Verification items for the finished model (mm, model axes). Face numbers are marked on the shaded views. A direction names the side the tool comes from. Coordinates: 2 decimals unless noted, no trailing zeros. Order: outer loops, then holes, each group sorted by start corner. A loop starts at its lowest first (then second) coordinate and runs counter-clockwise, first axis right, second up. Notation, with made-up numbers: M -24.75,-40 L 13.25,-40 A13 ccw 13.25,-36 Z; hole C 47,60 d6. An arc over 180 degrees is marked long. Write item = value, one per line.
Autodesk Inventor part; units mm, degrees
ref_plane "YZ Plane" through (0, 0, 0) normal (1, 0, 0) x (0, 1, 0)
ref_plane "XZ Plane" through (0, 0, 0) normal (0, 1, 0) x (-1, 0, 0)
ref_plane "XY Plane" through (0, 0, 0) normal (0, 0, 1) x (1, 0, 0)
sketch "Sketch1" plane through (0, 0, 0) normal (1, 0, 0) x (0, 1, 0)
  line L0 (-6, -12.5) -> (-6, -12.9)
  arc A0 (-6, -12.9) -> (-5.6, -13.3) centre (-5.6, -12.9) ccw
  line L1 (-5.6, -13.3) -> (-4.9, -13.3)
  arc A1 (-4.9, -13.3) -> (-4.7, -13.1) centre (-4.9, -13.1) ccw
  line L2 (-4.7, -13.1) -> (-4.7, -12.85)
  arc A2 (-4.5, -12.65) -> (-4.7, -12.85) centre (-4.5, -12.85) ccw
  line L3 (-4.5, -12.65) -> (-1.8, -12.65)
  arc A3 (-1.4, -13.05) -> (-1.8, -12.65) centre (-1.8, -13.05) ccw
  line L4 (-1.4, -13.05) -> (-1.4, -18.75)
  line L5 (-1.8, -19.15) -> (-4.5, -19.15)
  arc A4 (-1.8, -19.15) -> (-1.4, -18.75) centre (-1.8, -18.75) ccw
  arc A5 (-4.7, -18.95) -> (-4.5, -19.15) centre (-4.5, -18.95) ccw
  line L6 (-4.7, -18.95) -> (-4.7, -18.7)
  arc A6 (-4.7, -18.7) -> (-4.9, -18.5) centre (-4.9, -18.7) ccw
  line L7 (-4.9, -18.5) -> (-5.6, -18.5)
  arc A7 (-5.6, -18.5) -> (-6, -18.9) centre (-5.6, -18.9) ccw
  line L8 (-6, -18.9) -> (-6, -19.5)
  line L9 (-6.5, -6.5) -> (-6.5, -12.5)
  line L10 (-6.5, -12.5) -> (-2.5, -12.5)
  line L11 (-1.05, -19.5) -> (-6.5, -19.5)
  line L12 (-6.5, -19.5) -> (-6.5, -26)
  line L13 (-6.5, -26) -> (-1.05, -26)
  line L14 (-6, -26) -> (-6, -26.6)
  arc A8 (-6, -26.6) -> (-5.6, -27) centre (-5.6, -26.6) ccw
  line L15 (-5.6, -27) -> (-4.9, -27)
  arc A9 (-4.9, -27) -> (-4.7, -26.8) centre (-4.9, -26.8) ccw
  arc A10 (-4.5, -26.35) -> (-4.7, -26.55) centre (-4.5, -26.55) ccw
  line L16 (-4.7, -26.8) -> (-4.7, -26.55)
  line L17 (-4.5, -26.35) -> (-1.8, -26.35)
  arc A11 (-1.4, -26.75) -> (-1.8, -26.35) centre (-1.8, -26.75) ccw
  line L18 (-1.4, -26.75) -> (-1.4, -32.45)
  arc A12 (-1.8, -32.85) -> (-1.4, -32.45) centre (-1.8, -32.45) ccw
  line L19 (-1.8, -32.85) -> (-4.5, -32.85)
  arc A13 (-4.7, -32.65) -> (-4.5, -32.85) centre (-4.5, -32.65) ccw
  line L20 (-4.7, -32.65) -> (-4.7, -32.4)
  arc A14 (-4.7, -32.4) -> (-4.9, -32.2) centre (-4.9, -32.4) ccw
  line L21 (-4.9, -32.2) -> (-5.6, -32.2)
  arc A15 (-5.6, -32.2) -> (-6, -32.6) centre (-5.6, -32.6) ccw
  line L22 (-6, -32.6) -> (-6, -33)
  line L23 (-2.5, -33) -> (-6.5, -33)
  line L24 (-6.5, -33) -> (-6.5, -39)
  line L25 (32.5, 0) -> (0, 0)
  circle A16 centre (0, -6.5) radius 4.75
  circle A17 centre (32.5, -6.5) radius 4.75
  circle A18 centre (0, -39) radius 4.75
  circle A19 centre (32.5, -39) radius 4.75
  line L26 (39, -26) -> (39, -19.5)
  line L27 (39, -12.5) -> (39, -6.5)
  line L28 (39, -39) -> (39, -33)
  line L29 (26.5, -45.5) -> (32.5, -45.5)
  line L30 (0, -45.5) -> (6, -45.5)
  line L31 (13, -45.5) -> (19.5, -45.5)
  circle A20 centre (16.25, -22.75) radius 15
  circle A21 centre (16.2588, 5.0016) radius 2.5
  circle A22 centre (16.25, -50.5) radius 2.5
  circle A23 centre (16.25, -22.75) radius 5
  circle A24 centre (16.25, -22.75) radius 8.45
  line L32 (24.75, -27.6575) -> (24.75, -17.8425)
  line L33 (44, 10) -> (-11.5, 10)
  line L34 (-11.5, 10) -> (-11.5, -55.5)
  line L35 (-11.5, -55.5) -> (44, -55.5)
  line L36 (44, -55.5) -> (44, 10)
  line L37 (-11.5, 30) -> (44, 30)
  line L38 (-11.5, -75.5) -> (-11.5, 30)
  line L39 (44, 30) -> (44, -75.5)
  line L40 (44, -75.5) -> (-11.5, -75.5)
  circle A25 centre (16.25, -65.5) radius 5
  circle A26 centre (16.25, 20) radius 5
  line L41 (44, 30) -> (44, 50)
  line L42 (44, -75.5) -> (44, -95.5)
  line L43 (110, 50) -> (84, 50)
  line L44 (84, 50) -> (84, -95.5)
  line L45 (84, -95.5) -> (110, -95.5)
  line L46 (110, -95.5) -> (110, 50)
  line L47 (84, 50) -> (104, 50)
  line L48 (104, -95.5) -> (84, -95.5)
  line L49 (84, -95.5) -> (84, 50)
  line L50 (84, 50) -> (64, 50)
  line L51 (64, 50) -> (64, -95.5)
  line L52 (64, -95.5) -> (84, -95.5)
  line L53 (84, -95.5) -> (84, 50)
  line L54 (64, 50) -> (44, 50)
  line L55 (44, 50) -> (44, -95.5)
  line L56 (44, -95.5) -> (64, -95.5)
  line L57 (64, -95.5) -> (64, 50)
  line L58 (44, 30) -> (54, 30)
  line L59 (100.8097, 50) -> (100.8097, 40)
  line L60 (94, -95.5) -> (94, -85.5)
  line L61 (110, 40) -> (54, 40)
  line L62 (54, 40) -> (54, -85.5)
  line L63 (54, -85.5) -> (110, -85.5)
  line L64 (110, 50) -> (136, 50)
  line L65 (136, 50) -> (136, 40)
  line L66 (136, 40) -> (110, 40)
  line L67 (110, -85.5) -> (136, -85.5)
  line L68 (136, -85.5) -> (136, -95.5)
  line L69 (136, -95.5) -> (110, -95.5)
  dimension "d0" = 20
  dimension "d1" = 20
  dimension "d2" = 55.5
  dimension "d3" = 26
  dimension "d5" = 20
  dimension "d6" = 45.5
  dimension "d7" = 20
  dimension "d8" = 10
  dimension "d9" = 10
  dimension "d10" = 26
extrude "Extrusion1" add sketch "Sketch1" along normal blind 75.5 contours L39 L58 L62 L63 L51 L56 L42 L36 | L41 L54 L51 L61 L62 L58 | L50 L44 L61 L51 | L51 L63 L44 L52 | L43 L59 L61 L44 | L44 L63 L60 L45 | L43 L46 L61 L59 | L60 L63 L46 L45 | L64 L65 L66 L46 | L67 L68 L69 L46
sketch "Sketch2" plane through (0, 44, -95.5) normal (0, -1, 0) x (1, 0, 0)
  line L0 (15.5, 83) -> (15.5, 82.6)
  arc A0 (15.5, 82.6) -> (15.9, 82.2) centre (15.9, 82.6) ccw
  line L1 (15.9, 82.2) -> (16.6, 82.2)
  arc A1 (16.6, 82.2) -> (16.8, 82.4) centre (16.6, 82.4) ccw
  line L2 (16.8, 82.4) -> (16.8, 82.65)
  arc A2 (17, 82.85) -> (16.8, 82.65) centre (17, 82.65) ccw
  line L3 (17, 82.85) -> (19.7, 82.85)
  arc A3 (20.1, 82.45) -> (19.7, 82.85) centre (19.7, 82.45) ccw
  line L4 (20.1, 82.45) -> (20.1, 76.75)
  line L5 (19.7, 76.35) -> (17, 76.35)
  arc A4 (19.7, 76.35) -> (20.1, 76.75) centre (19.7, 76.75) ccw
  arc A5 (16.8, 76.55) -> (17, 76.35) centre (17, 76.55) ccw
  line L6 (16.8, 76.55) -> (16.8, 76.8)
  arc A6 (16.8, 76.8) -> (16.6, 77) centre (16.6, 76.8) ccw
  line L7 (16.6, 77) -> (15.9, 77)
  arc A7 (15.9, 77) -> (15.5, 76.6) centre (15.9, 76.6) ccw
  line L8 (15.5, 76.6) -> (15.5, 76)
  line L9 (15, 89) -> (15, 83)
  line L10 (15, 83) -> (19, 83)
  line L11 (20.45, 76) -> (15, 76)
  line L12 (15, 76) -> (15, 69.5)
  line L13 (15, 69.5) -> (20.45, 69.5)
  line L14 (15.5, 69.5) -> (15.5, 68.9)
  arc A8 (15.5, 68.9) -> (15.9, 68.5) centre (15.9, 68.9) ccw
  line L15 (15.9, 68.5) -> (16.6, 68.5)
  arc A9 (16.6, 68.5) -> (16.8, 68.7) centre (16.6, 68.7) ccw
  arc A10 (17, 69.15) -> (16.8, 68.95) centre (17, 68.95) ccw
  line L16 (16.8, 68.7) -> (16.8, 68.95)
  line L17 (17, 69.15) -> (19.7, 69.15)
  arc A11 (20.1, 68.75) -> (19.7, 69.15) centre (19.7, 68.75) ccw
  line L18 (20.1, 68.75) -> (20.1, 63.05)
  arc A12 (19.7, 62.65) -> (20.1, 63.05) centre (19.7, 63.05) ccw
  line L19 (19.7, 62.65) -> (17, 62.65)
  arc A13 (16.8, 62.85) -> (17, 62.65) centre (17, 62.85) ccw
  line L20 (16.8, 62.85) -> (16.8, 63.1)
  arc A14 (16.8, 63.1) -> (16.6, 63.3) centre (16.6, 63.1) ccw
  line L21 (16.6, 63.3) -> (15.9, 63.3)
  arc A15 (15.9, 63.3) -> (15.5, 62.9) centre (15.9, 62.9) ccw
  line L22 (15.5, 62.9) -> (15.5, 62.5)
  line L23 (19, 62.5) -> (15, 62.5)
  line L24 (15, 62.5) -> (15, 56.5)
  line L25 (54, 95.5) -> (21.5, 96.1203)
  circle A16 centre (21.5, 89) radius 4.75
  circle A17 centre (54, 89) radius 4.75
  circle A18 centre (21.5, 56.5) radius 4.75
  circle A19 centre (54, 56.5) radius 4.75
  line L26 (60.5, 69.5) -> (60.5, 76)
  line L27 (60.5, 83) -> (60.5, 89)
  line L28 (60.5, 56.5) -> (60.5, 62.5)
  line L29 (48, 50) -> (54, 50)
  line L30 (21.5, 50) -> (27.5, 50)
  line L31 (34.5, 50) -> (41, 50)
  circle A20 centre (37.75, 72.75) radius 15
  circle A21 centre (37.7588, 100.5016) radius 2.5
  circle A22 centre (37.75, 45) radius 2.5
  circle A23 centre (37.75, 72.75) radius 5
  circle A24 centre (37.75, 72.75) radius 8.45
  line L32 (46.25, 67.8425) -> (46.25, 77.6575)
  line L33 (65.5, 105.5) -> (10, 105.5)
  line L34 (10, 105.5) -> (10, 40)
  line L35 (10, 40) -> (65.5, 40)
  line L36 (65.5, 40) -> (65.5, 105.5)
  line L37 (10, 125.5) -> (65.5, 125.5)
  line L38 (10, 20) -> (10, 125.5)
  line L39 (65.5, 125.5) -> (65.5, 20)
  line L40 (65.5, 20) -> (10, 20)
  circle A25 centre (37.75, 30) radius 5
  circle A26 centre (37.75, 115.5) radius 5
  line L41 (0, 145.5) -> (0, 0)
  line L42 (75.5, 145.5) -> (75.5, 0)
  line L43 (0, 145.5) -> (75.5, 0)
  line L44 (75.5, 0) -> (75.5, 145.5)
  line L45 (75.5, 145.5) -> (0, 0)
  line L46 (37.75, 72.75) -> (-23.5643, 72.75)
  point P0 (0, 95.5)
extrude "Extrusion2" cut sketch "Sketch2" against normal blind 75.5 contours A25 | A26
sketch "Sketch3" plane through (0, 44, -95.5) normal (0, 0, -1) x (-1, 0, 0)
  line L0 (0, 92) -> (-75.5, 92)
  line L1 (-75.5, 92) -> (-10, 92)
  line L2 (-10, 92) -> (-10, 36.5)
  line L3 (-10, 36.5) -> (-75.5, 36.5)
  line L4 (-75.5, 36.5) -> (-75.5, 92)
  line L5 (-42.75, 36.5) -> (-42.75, 92)
  line L6 (-10, 36.5) -> (-42.75, 92)
  line L7 (-26.375, 64.25) -> (-42.75, 64.25)
  line L8 (-42.75, 36.5) -> (-75.5, 92)
  line L9 (-59.125, 64.25) -> (-42.75, 64.25)
  circle A0 centre (-26.375, 64.25) radius 5
  circle A1 centre (-59.125, 64.25) radius 5
  point P0 (0, -44)
  dimension "d21" = 65.5
  dimension "d22" = 55.5
  dimension "d23" = 10
  dimension "d24" = 10
extrude "Extrusion3" cut sketch "Sketch3" against normal through all contours A0 L6 | L6 L7 A0 | A0 L7 L6 | A1 L9 L8 | L8 A1 | A1 L8 L9
sketch "Sketch4" plane through (0, 44, -95.5) normal (0, 0, -1) x (-1, 0, 0)
  line L0 (0, 0) -> (-75.5, 0)
  line L1 (-75.5, 10) -> (-75.5, 92)
  line L2 (0, 0) -> (-75.5, 0)
  line L3 (-75.5, 0) -> (-75.5, 18.25)
  line L4 (-75.5, 18.25) -> (0, 18.25)
  line L5 (0, 18.25) -> (0, 0)
  line L6 (0, 92) -> (-75.5, 92)
  line L7 (0, 18.25) -> (-75.5, 18.25)
  line L8 (-75.5, 18.25) -> (-75.5, 92)
  line L9 (-75.5, 92) -> (0, 92)
  line L10 (0, 92) -> (0, 18.25)
  point P0 (0, -44)
  dimension "d27" = 18.25
extrude "Extrusion4" cut sketch "Sketch4" against normal through all contours L4 L1 L6 L10
sketch "Sketch5" plane through (75.5, 44, -95.5) normal (0, 0, -1) x (-1, 0, 0)
  line L0 (0, 18.25) -> (75.5, 18.25)
  line L1 (0, 0) -> (0, 18.25)
  line L2 (75.5, 18.25) -> (0, 18.25)
  line L3 (0, 18.25) -> (0, 13.25)
  line L4 (0, 13.25) -> (75.5, 13.25)
  line L5 (75.5, 13.25) -> (75.5, 18.25)
  point P0 (75.5, -44)
  dimension "d30" = 5
sketch "Sketch6" plane through (0, 44, 50) normal (0, 0, 1) x (1, 0, 0)
  line L0 (75.5, 18.25) -> (75.5, 10)
  line L1 (0, 18.25) -> (0, 0)
  line L2 (75.5, 18.25) -> (0, 18.25)
  line L3 (0, 18.25) -> (0, 13.25)
  line L4 (0, 13.25) -> (75.5, 13.25)
  line L5 (75.5, 13.25) -> (75.5, 18.25)
  point P0 (0, -44)
  dimension "d31" = 5
extrude "Extrusion5" add sketch "Sketch6" along normal blind 20
extrude "Extrusion6" add sketch "Sketch5" along normal blind 20
sketch "Sketch7" plane through (0, 57.25, -95.5) normal (0, -1, 0) x (1, 0, 0)
  line L0 (0, 10) -> (0, -20)
  line L1 (0, 0) -> (75.5, 0)
  line L2 (0, -20) -> (75.5, 0)
  line L3 (75.5, 0) -> (37.75, -10)
  line L4 (37.75, -10) -> (37.75, -2.094)
  line L5 (0, 145.5) -> (0, 165.5)
  line L6 (75.5, 145.5) -> (75.5, 165.5)
  line L7 (0, 145.5) -> (75.5, 165.5)
  line L8 (75.5, 165.5) -> (37.75, 159.321)
  line L9 (37.75, 159.321) -> (37.75, 155.5)
  circle A0 centre (37.75, -10) radius 5
  circle A1 centre (37.75, 155.5) radius 5
  point P0 (0, 95.5)
  dimension "d36" = 10
  dimension "d37" = 10
extrude "Extrusion7" cut sketch "Sketch7" against normal blind 20 contours A0 L4 L2 | L2 A0 | L2 L4 A0 | A1 L8 L9 L7 | L7 A1 | L9 L8 A1 L7
properties part number "CarroSuperior"
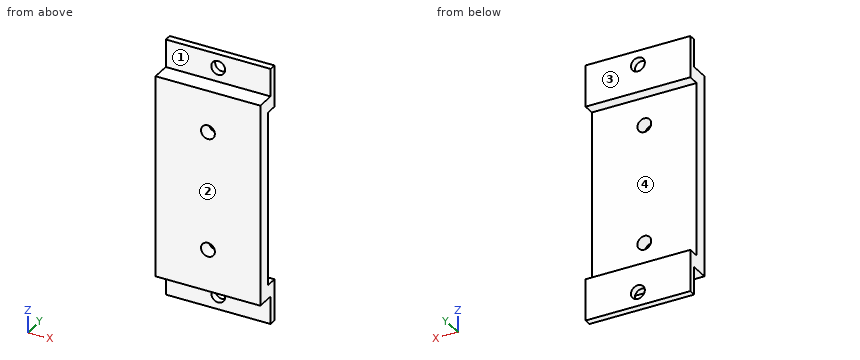
Item 1: Sectioned sample at D-D, the plane x = 22. Enter the section's corners in (y, z).
Report:
outline = M 44,-95.5 L 57.25,-95.5 L 57.25,-115.5 L 62.25,-115.5 L 62.25,-85.5 L 54,-85.5 L 54,40 L 62.25,40 L 62.25,70 L 57.25,70 L 57.25,50 L 44,50 Z
Item 2: Gauge pin test, flat ends, axial feed: pin 1 (6 mm diameter, centred on x = 37.75, z = -105.5, fed in from -Y); pin 2 (4 mm diameter, centred on x = 13.5, z = -1.5, fed in from +Y); pin 3 (10.5 mm diameter, centred on x = 52, y = 50.5, fed in from -Z); pin 4 (4 mm diameter, centred on x = 23, y = 51.5, fed in from +Z). Record the tip position at first contact, or that the pin passes through.
Report:
pin_1 = through
pin_2 = 54
pin_3 = -95.5
pin_4 = 50
Item 3: Release check for a two-part mould opening along Z. For the marked faces 3 and 4 record: pulls with the +Z half, pulls with the -Z half, needs draft (parallel to the pull), parting line crosses it, or undercut.
Report:
face_3 = needs draft
face_4 = undercut
Item 4: Scan lines: L1, parallel to Z at x = 37.75, y = 60.4; L2, parallel to X at y = 59.85, z = -105.5; L3, parallel to Z at x = 71, y = 57. Record each from-to range of solid material in increasing order. Write a range as from..to.
Report:
L1 = -115.5..-110.5, -100.5..-85.5, 40..55, 65..70
L2 = 0..32.75, 42.75..75.5
L3 = -95.5..-85.5, 40..50
Item 5: Tool access check on the marked faces 1 and 2. Record the directions out of +Z, -Z, +X, -X, +Y, -Y that give a thin tool (end or side, any length) a straight path to the whole face; none if there is none.
Report:
face_1 = +Z, +X, -X, -Y
face_2 = +Z, -Z, +X, -X, -Y
Item 6: Sectioned sample at B-B, the plane x = 37.75. Enter the section's corners in (y, z).
Report:
outline = M 44,-95.5 L 57.25,-95.5 L 57.25,-100.5 L 62.25,-100.5 L 62.25,-85.5 L 54,-85.5 L 54,-70.5 L 44,-70.5 Z; M 44,-60.5 L 54,-60.5 L 54,15 L 44,15 Z; M 44,25 L 54,25 L 54,40 L 62.25,40 L 62.25,55 L 57.25,55 L 57.25,50 L 44,50 Z; M 57.25,-115.5 L 62.25,-115.5 L 62.25,-110.5 L 57.25,-110.5 Z; M 57.25,65 L 62.25,65 L 62.25,70 L 57.25,70 Z
Item 7: Sectioned sample at C-C, the plane z = -105.5. Enter the section's corners in (x, y), then the cut area to 4 significant figures.
Report:
outline = M 0,57.25 L 32.75,57.25 L 32.75,62.25 L 0,62.25 Z; M 42.75,57.25 L 75.5,57.25 L 75.5,62.25 L 42.75,62.25 Z
area = 327.5 mm^2
Item 8: Sectioned sample at A-A, the plane y = 60.25. Enter the section's corners in (x, z), then the cut area to 3 significant figures.
Report:
outline = M 0,-115.5 L 75.5,-115.5 L 75.5,-85.5 L 0,-85.5 Z; M 0,40 L 75.5,40 L 75.5,70 L 0,70 Z; hole C 37.75,-105.5 d10; hole C 37.75,60 d10
area = 4,370 mm^2
